Verification items for the finished model (mm, model axes). A direction names the side the tool comes from. Round coordinates to 2 decimals unless told otherwise and drop trailing zeros. Order: outer loops, then holes, each group sorted by start corner. A loop starts at its lowest first (then second) coordinate and runs counter-clockwise, first axis right, second up.
```python
from build123d import *

# Parameters (mm, degrees)
ESQUISSE2_R             = 92.5
ENL_V_MAT_EXTRU_1_DEPTH = 96.765338197
ESQUISSE6_R             = 5
ESQUISSE6_R_2           = 4
ENL_V_MAT_EXTRU_2_DEPTH = 96.765338197
ESQUISSE7_R             = 2.5
ENL_V_MAT_EXTRU_3_DEPTH = 96.765338197


with BuildPart() as part:
    # Esquisse1 → Base-Révolution (revolve)
    with BuildSketch(Plane.XY, mode=Mode.PRIVATE) as base_r_volution_sk:
        Polygon((0, 24), (0, 28), (12, 28), (12, 59), (29, 59), (29, 22.5), (59, 22.5), (59, 12), (19, 12), (19, 24), align=None)
    revolve(base_r_volution_sk.sketch.rotate(Axis((-50, 0, 0), (1, 0, 0)), 90), axis=Axis((-50, 0, 0), (1, 0, 0)))

    # Esquisse2 → Enlèv. mat.-Extru.1 (cut, through all)
    with BuildSketch(Plane.ZY.offset(-12)):
        with Locations((0, 125)):
            Circle(ESQUISSE2_R)
    extrude(amount=-ENL_V_MAT_EXTRU_1_DEPTH, mode=Mode.SUBTRACT)

    # Esquisse6 → Enlèv. mat.-Extru.2 (cut, through all)
    with BuildSketch(Plane.ZY.offset(-12)):
        with Locations((0, -35)):
            Circle(ESQUISSE6_R)
        with Locations((0, -50)):
            Circle(ESQUISSE6_R_2)
    extrude(amount=-ENL_V_MAT_EXTRU_2_DEPTH, mode=Mode.SUBTRACT)

    # Esquisse7 → Enlèv. mat.-Extru.3 (cut, through all)
    with BuildSketch(Plane.ZY.offset(-12)):
        with Locations((-26, 26)):
            Circle(ESQUISSE7_R)
        with Locations((26, -26)):
            Circle(ESQUISSE7_R)
    extrude(amount=-ENL_V_MAT_EXTRU_3_DEPTH, mode=Mode.SUBTRACT)


solid = part.part
```
1) Sectioned sample at A-A on x = 25. Record the cut outline in (y, z), then the cut area to 3 significant figures.
2) Draft check along Y on faces 4 (the flat face through (0, -13, -21)), 5 (the cylindrical face through (6.08, 24.84, 12.92)), 6 (the flat face through (19, -6, 11)). Enter one of: released by +Y, released by -Y, zero draft, split by the parting line, or undercut.
3) Scan lines: probe 1 along Y at (x, z) = (21, 0); probe 2 along Y at (x, z) = (11, 0); probe 3 along Y at (x, z) = (18.25, 0). Record each from-to range of solid material in increasing order.
4) Tool access check on faces 1 (the cylindrical face through (20.38, 28.48, -26.33)), 2 (the cylindrical face through (44.21, 19.961, 10.382)), 3 (the cylindrical face through (9.37, -7.21, 22.89)). Record the directions out of +Z, -Z, +X, -X, +Y, -Y that give a thin tool (end or side, any length) a straight path to the whole face; none if there is none.
5) Sectioned sample at B-B on y = 0. Record the cut outline in (x, z), then the cut area to 3 significant figures.
6) Sectioned sample at C-C on z = -26. Record the cut outline in (x, y), then the cut area to 3 significant figures.
7) Sectioned sample at D-D on x = 4.5. Record the cut outline in (y, z), then the cut area to 3 significant figures.
8) Go/stop test with flat-tipped pins: pin 1 Ø5 at (y, z) = (-45.5, -26.5) entering from +X; pin 2 Ø8 at (x, z) = (25.5, 34) entering from -Y; pin 3 Ø3 at (x, z) = (15, 0.5) entering from -Y; pin 4 Ø9 at (y, z) = (-50, 0) entering from -X. Record where each tip stops, or that it passes through.
Returned:
1. outline: (42.2, -41.23) arc R92.5 cw to (42.2, 41.23) arc R59 ccw (long way) to start; hole circle Ø8 at (-50, 0); hole circle Ø10 at (-35, 0); hole circle Ø5 at (-26, 26); hole circle Ø24 at (0, 0); hole circle Ø5 at (26, -26)
1. area: 8,820 mm2
2. face 4: zero draft
2. face 5: split by the parting line
2. face 6: undercut
3. probe 1: y = -59 to -54, -46 to -40, -30 to -12, 12 to 32.5
3. probe 2: y = -28 to -24, 24 to 28
3. probe 3: y = -59 to -54, -46 to -40, -30 to -24, 24 to 32.5
4. face 1: +X, -X
4. face 2: +X
4. face 3: -X
5. outline: (0, -28) - (12, -28) - (12, -59) - (29, -59) - (29, -22.5) - (59, -22.5) - (59, -12) - (19, -12) - (19, -24) - (0, -24) - close; (0, 24) - (19, 24) - (19, 12) - (59, 12) - (59, 22.5) - (29, 22.5) - (29, 59) - (12, 59) - (12, 28) - (0, 28) - close
5. area: 2,160 mm2
6. outline: (0, -10.39) - (12, -10.39) - (12, -52.96) - (29, -52.96) - (29, 23.5) - (12, 23.5) - (12, 10.39) - (0, 10.39) - close; (12, 28.5) - (29, 28.5) - (29, 36.23) - (12, 36.23) - close
6. area: 1,680 mm2
7. outline: circle Ø56 at (0, 0); hole circle Ø48 at (0, 0)
7. area: 653 mm2
8. pin 1: stops at x = 29
8. pin 2: stops at y = -50.8
8. pin 3: stops at y = -59
8. pin 4: stops at x = 12
